```python
from build123d import *

# Parameters (mm, degrees)
SKETCH1_R           = 1.65
BOSS_EXTRUDE1_DEPTH = 4
SKETCH2_R           = 4
SKETCH2_R_2         = 1.65
BOSS_EXTRUDE2_DEPTH = 3.5


with BuildPart() as part:
    # Sketch1 → Boss-Extrude1 (new body)
    with BuildSketch(Plane.XY):
        with BuildLine():
            Line((-25, 4), (0, 4))
            ThreePointArc((0, 4), (4, 0), (0, -4))
            Line((0, -4), (-25, -4))
            ThreePointArc((-25, -4), (-29, 0), (-25, 4))
        make_face()
        Circle(SKETCH1_R, mode=Mode.SUBTRACT)
        with Locations((-25, 0)):
            Circle(SKETCH1_R, mode=Mode.SUBTRACT)
    extrude(amount=BOSS_EXTRUDE1_DEPTH)

    # Sketch2 → Boss-Extrude2 (add)
    with BuildSketch(Plane.XY.offset(4)):
        with Locations(Location((-25, 0, 0), (0, 0, 270))):
            Circle(SKETCH2_R)
        with Locations((-25, 0)):
            Circle(SKETCH2_R_2, mode=Mode.SUBTRACT)
    extrude(amount=BOSS_EXTRUDE2_DEPTH)


solid = part.part
```
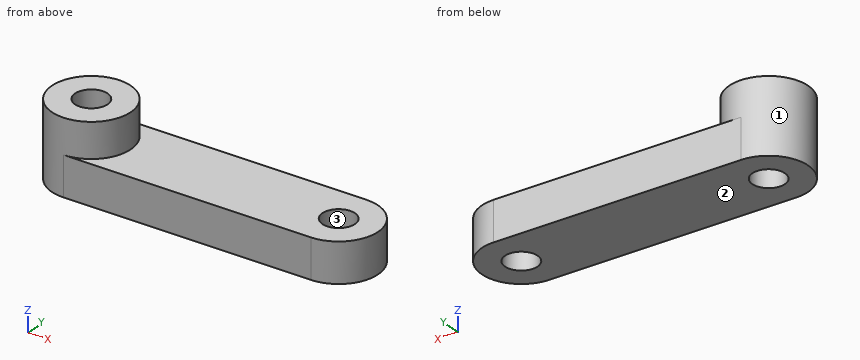
Could you check a few things on this model? Use its own coordinates, in mm. Face numbers are marked on the shaded views. Give positions to 0.01 mm unless a question says otherwise; leave off trailing zeros. Loops run counter-clockwise (first coordinate to the right, second up) from the corner with the lowest first, then second, coordinate; pieces in that order, holes last. Notation, with made-up numbers: (23, -23.5) - (50, -23.5) arc R13 cw to (50, -4.5) - close; hole circle Ø7 at (18, 0.25). An arc over 180 degrees is marked (long way). Answer in a Markdown table with one row per item. Add a question column.
Q1. If we section it at C-C (x = -26): List the corners of the cut face in (y, z) for me.
Q2. For pin 1 (2 mm diameter, centred on y = -3, z = 1, fed in from +X); pin 2 (3 mm diameter, centred on x = 0, y = 0, fed in from -Z); pin 3 (4 mm diameter, centred on x = -5, y = -1.5, fed in from +Z); pin 4 (2 mm diameter, centred on y = -2, z = 4, fed in from +X), each with a flat end and sliding along its axis, tell me the tip position at first contact or that it passes through.
Q3. If we section it at D-D (x = -16): List the corners of the cut face in (y, z) for me, plus the area to 3 significant figures.
Q4. We'd pull the mould along X, two halves only. Please class the marked faces 1, 2 and 3: +X half, -X half, draft (parallel to the pull), parting line (faces both ways), or undercut.
Q5. If we section it at B-B (z = 4.75): List the corners of the cut face in (x, y) for me, plus the area to 3 significant figures.
Q6. If we section it at A-A (y = 0): List the corners of the cut face in (x, z) for me, plus the area to 3 significant figures.
Q7. Please list where these lines run through material, in increasing order: L1, parallel to Y at x = -25, z = 2; L2, parallel to Z at x = -21, y = 2.75; L3, parallel to X at y = 0.25, z = 3.5. Write a range as from..to.
The answers:
| question | item | result |
|---|---|---|
| 1 | outline | (-3.87, 0) - (-1.31, 0) - (-1.31, 7.5) - (-3.87, 7.5) - close; (1.31, 0) - (3.87, 0) - (3.87, 7.5) - (1.31, 7.5) - close |
| 2 | pin 1 | stops at x = 3.46 |
| 2 | pin 2 | passes through |
| 2 | pin 3 | stops at z = 4 |
| 2 | pin 4 | stops at x = 3.87 |
| 3 | outline | (-4, 0) - (4, 0) - (4, 4) - (-4, 4) - close |
| 3 | area | 32.0 mm^2 |
| 4 | face 1 | parting line |
| 4 | face 2 | draft |
| 4 | face 3 | undercut |
| 5 | outline | circle Ø8 at (-25, 0); hole circle Ø3.3 at (-25, 0) |
| 5 | area | 41.7 mm^2 |
| 6 | outline | (-29, 0) - (-26.65, 0) - (-26.65, 7.5) - (-29, 7.5) - close; (-23.35, 0) - (-1.65, 0) - (-1.65, 4) - (-21, 4) - (-21, 7.5) - (-23.35, 7.5) - close; (1.65, 0) - (4, 0) - (4, 4) - (1.65, 4) - close |
| 6 | area | 122 mm^2 |
| 7 | L1 | y = -4..-1.65, 1.65..4 |
| 7 | L2 | z = 0..4 |
| 7 | L3 | x = -28.99..-26.63, -23.37..-1.63, 1.63..3.99 |
